Part model, mm, in its own coordinate system. A direction names the side the tool comes from. Coordinates: 2 decimals unless noted, no trailing zeros. Loops run counter-clockwise (first coordinate to the right, second up) from the corner with the lowest first, then second, coordinate; pieces in that order, holes last. Notation, with made-up numbers: M 12,42 L 34,42 A16 cw 34,60 Z; hole C -1.5,85.5 d11. An arc over 180 degrees is marked long. Answer as a JSON object with one key per item and string values. Group by question number.
1. Saw through at D-D on y = -69.85. Write the cut outline in (x, z), then the cut area to 3 significant figures.
2. Saw through at B-B on z = 59.5. Write the cut outline in (x, y) (3 decimals).
3. Saw through at A-A on y = -50.5. Write the cut outline in (x, z), then the cut area to 3 significant figures.
4. Mould opens along X. For faces 4 (the face through (-116.715, -59, 40)), 5 (the face through (134.11, -27, 39)), 6 (the face through (2, -27, -36.221)), 7 (the face through (67, -31, -26.696)) say: released by +X, released by -X, zero draft, split by the parting line, or undercut.
5. Saw through at C-C on x = -52.5. Write the cut outline in (y, z) (3 decimals), then the cut area to 3 significant figures.
6. Drop flat-ended pins along their axis: pin 1 Ø18 at (x, z) = (-35, 84) entering from -Y (3 decimals); pin 2 Ø3 at (y, z) = (-60, 41.5) entering from -X; pin 3 Ø3 at (y, z) = (-58, 41.5) entering from +X. Give the stop position or say it passes through.
7. 3-axis set-ups, long thin cutter, end or side, ignore diameter. For faces 1 (the face through (-126.24, -27, 41)), 2 (the face through (-34.16, -69.56, 40.07)), 3 (the face through (-116.715, -31, 3)): which of +Z, -Z, +X, -X, +Y, -Y reach the whole face in a straight line?
8. Drill centre lines: L1, parallel to Z at x = 55, y = -53; L2, parallel to X at y = -44, z = 47.5; L3, parallel to Y at x = 6.5, z = 43 (3 decimals). Where is each one in solid material? Low to high.
from build123d import *

# Parameters (mm, degrees)
F0_W     = 260.35
F0_H     = 152.4
F1_DEPTH = 9.525
F3_DEPTH = 44.45
F5_DEPTH = 88.9
F7_D     = 25.4
F9_DEPTH = 25.4


with BuildPart() as f1:
    # F0 (on Front) → F1 (new body)
    with BuildSketch(Plane.XZ):
        with Locations((3.93492, 39.978574)):
            Rectangle(F0_W, F0_H)
    extrude(amount=F1_DEPTH)

    # F2 (on face) → F3 (join)
    with BuildSketch(Plane.XZ.offset(9.525)):
        Polygon((-126.24008, 106.653574), (-126.24008, -26.696426), (-116.71508, -26.696426), (-116.71508, 49.017824), (-116.71508, 106.653574), align=None)
        Polygon((124.58492, 106.653574), (134.10992, 106.653574), (134.10992, 116.178574), (-126.24008, 116.178574), (-126.24008, 106.653574), (-116.71508, 106.653574), (-0.82758, 106.653574), (8.69742, 106.653574), align=None)
        Polygon((-0.82758, -26.696426), (8.69742, -26.696426), (8.69742, 55.01255), (8.69742, 106.653574), (-0.82758, 106.653574), (-0.82758, 77.835699), align=None)
        Polygon((124.58492, -26.696426), (134.10992, -26.696426), (134.10992, 106.653574), (124.58492, 106.653574), (124.58492, 65.446369), align=None)
        Polygon((-126.24008, -36.221426), (134.10992, -36.221426), (134.10992, -26.696426), (124.58492, -26.696426), (8.69742, -26.696426), (-0.82758, -26.696426), (-116.71508, -26.696426), (-126.24008, -26.696426), align=None)
    extrude(amount=F3_DEPTH)

    # F4 (on face) → F5 (join)
    with BuildSketch(Plane.XZ.offset(9.525)):
        Polygon((-116.71508, 33.628574), (38.57762, 33.628574), (124.58492, 33.628574), (124.58492, 46.328574), (37.81344, 46.328574), (-4.043767, 46.328574), (-116.71508, 46.328574), align=None)
    extrude(amount=F5_DEPTH)

    # F7 (through all)
    with Locations(Plane(origin=(0, 0, 33.628574), x_dir=(1, 0, 0), z_dir=(0, 0, -1))):
        with Locations((-21.46508, 69.85), (-19.252239, 69.85), (-17.284498, 69.85), (-15.503385, 69.85), (-13.247554, 69.85), (-11.229082, 69.85), (-8.837353, 69.85), (-6.768152, 69.85), (-4.800411, 69.85), (-2.307222, 69.85), (-0.28875, 69.85), (1.628261, 69.85), (3.93492, 69.85), (5.801102, 69.85), (8.056932, 69.85), (10.68602, 69.85), (12.840387, 69.85), (14.85886, 69.85), (17.06396, 69.85), (19.218329, 69.85), (20.676916, 69.85), (23.255272, 69.85), (25.036385, 69.85), (26.868232, 69.85), (29.33492, 69.85)):
            Hole(F7_D / 2)

    # F8 (on face) → F9 (cut)
    with BuildSketch(Plane(origin=(0, 0, 33.628574), x_dir=(1, 0, 0), z_dir=(0, 0, -1))):
        with BuildLine():
            Line((-116.71508, 98.425), (-116.71508, 64.064013))
            ThreePointArc((-116.71508, 64.064013), (-79.559192, 76.709492), (-46.86508, 98.425))
            Line((-46.86508, 98.425), (-116.71508, 98.425))
        make_face()
        with BuildLine():
            Line((124.58492, 98.425), (54.73492, 98.425))
            ThreePointArc((54.73492, 98.425), (87.401467, 76.523831), (124.58492, 63.711519))
            Line((124.58492, 63.711519), (124.58492, 98.425))
        make_face()
    extrude(amount=-F9_DEPTH, mode=Mode.SUBTRACT)


solid = f1.part
Outcome:
{
 "1": {"outline": "M -95.82,33.63 L -34.17,33.63 L -34.17,46.33 L -95.82,46.33 Z; M 42.03,33.63 L 102.94,33.63 L 102.94,46.33 L 42.03,46.33 Z", "area": "1,560 mm²"},
 "2": {"outline": "M -126.24,-53.975 L -116.715,-53.975 L -116.715,-9.525 L -0.828,-9.525 L -0.828,-53.975 L 8.697,-53.975 L 8.697,-9.525 L 124.585,-9.525 L 124.585,-53.975 L 134.11,-53.975 L 134.11,0 L -126.24,0 Z"},
 "3": {"outline": "M -126.24,-36.22 L 134.11,-36.22 L 134.11,116.18 L -126.24,116.18 Z; hole M -116.72,-26.7 L -0.83,-26.7 L -0.83,33.63 L -116.72,33.63 Z; hole M -116.72,46.33 L -0.83,46.33 L -0.83,106.65 L -116.72,106.65 Z; hole M 8.7,-26.7 L 124.58,-26.7 L 124.58,33.63 L 8.7,33.63 Z; hole M 8.7,46.33 L 124.58,46.33 L 124.58,106.65 L 8.7,106.65 Z", "area": "11,700 mm²"},
 "4": {"face 4": "released by -X", "face 5": "released by +X", "face 6": "zero draft", "face 7": "undercut"},
 "5": {"outline": "M -93.761,33.629 L -9.525,33.629 L -9.525,-26.696 L -53.975,-26.696 L -53.975,-36.221 L 0,-36.221 L 0,116.179 L -53.975,116.179 L -53.975,106.654 L -9.525,106.654 L -9.525,46.329 L -93.761,46.329 Z", "area": "3,370 mm²"},
 "6": {"pin 1": "stops at y = -9.525", "pin 2": "stops at x = -116.72", "pin 3": "stops at x = 124.58"},
 "7": {"face 1": "+Z, -Z, -X, +Y, -Y", "face 2": "+Z, -Z", "face 3": "-Y"},
 "8": {"L1": "z = -36.22 to -26.7, 33.63 to 46.33, 106.65 to 116.18", "L2": "x = -126.24 to -116.72, -0.83 to 8.7, 124.58 to 134.11", "L3": "y = -98.425 to -82.531, -57.169 to 0"}
}
